from build123d import *

# Parameters (mm, degrees)
BOSS_EXTRUDE1_DEPTH  = 2.9
SOLENOID_PLACEMENT_W = 37.4
SOLENOID_PLACEMENT_H = 63.8
CUT_EXTRUDE1_DEPTH   = 103.571487266
CUT_EXTRUDE3_DEPTH   = 103.571487266
SKETCH4_W            = 13
SKETCH4_H            = 26.3
CUT_EXTRUDE4_DEPTH   = 98.286484159
CUT_EXTRUDE5_DEPTH   = 98.286484159
SKETCH6_R            = 2.25
CUT_EXTRUDE6_DEPTH   = 98.286484159


with BuildPart() as part:
    # Sketch1 → Boss-Extrude1 (new body)
    with BuildSketch(Plane(origin=(0, 0, 0), x_dir=(1, 0, 0), z_dir=(0, 1, 0))):
        with BuildLine():
            ThreePointArc((33.29110537, -64.404598464), (0, 72.5), (-33.29110537, -64.404598464))
            ThreePointArc((-33.29110537, -64.404598464), (0, -44.989799638), (33.29110537, -64.404598464))
        make_face()
    extrude(amount=BOSS_EXTRUDE1_DEPTH)

    # solenoid placement → Cut-Extrude1 (cut, through all)
    with BuildSketch(Plane(origin=(0, 2.9, 0), x_dir=(1, 0, 0), z_dir=(0, 1, 0))):
        with Locations((0, -3.8)):
            Rectangle(SOLENOID_PLACEMENT_W, SOLENOID_PLACEMENT_H)
    extrude(amount=-CUT_EXTRUDE1_DEPTH, mode=Mode.SUBTRACT)

    # Sketch3 → Cut-Extrude3 (cut, through all)
    with BuildSketch(Plane(origin=(0, 2.9, 0), x_dir=(1, 0, 0), z_dir=(0, 1, 0))):
        with BuildLine():
            Line((-34.63, -32.5), (-22.83, -32.5))
            Line((-22.83, -32.5), (-22.83, 32.5))
            Line((-22.83, 32.5), (-64.807406984, 32.5))
            ThreePointArc((-64.807406984, 32.5), (-72.5, 0), (-64.807406984, -32.5))
            Line((-64.807406984, -32.5), (-34.63, -32.5))
        make_face()
        with BuildLine():
            Line((34.63, -32.5), (64.807406984, -32.5))
            ThreePointArc((64.807406984, -32.5), (72.5, 0), (64.807406984, 32.5))
            Line((64.807406984, 32.5), (22.83, 32.5))
            Line((22.83, 32.5), (22.83, -32.5))
            Line((22.83, -32.5), (34.63, -32.5))
        make_face()
    extrude(amount=-CUT_EXTRUDE3_DEPTH, mode=Mode.SUBTRACT)

    # Sketch4 → Cut-Extrude4 (cut, through all)
    with BuildSketch(Plane(origin=(0, 2.9, 0), x_dir=(1, 0, 0), z_dir=(0, 1, 0))):
        with Locations((0, 41.25)):
            Rectangle(SKETCH4_W, SKETCH4_H)
    extrude(amount=-CUT_EXTRUDE4_DEPTH, mode=Mode.SUBTRACT)

    # Sketch5 → Cut-Extrude5 (cut, through all)
    with BuildSketch(Plane(origin=(0, 2.9, 0), x_dir=(1, 0, 0), z_dir=(0, 1, 0))):
        Polygon((-18.706882066, 48), (-21.853441033, 53.45), (-28.146558967, 53.45), (-31.293117934, 48), (-28.146558967, 42.55), (-21.853441033, 42.55), align=None)
        Polygon((21.853441033, 42.55), (18.706882066, 48), (21.853441033, 53.45), (28.146558967, 53.45), (31.293117934, 48), (28.146558967, 42.55), align=None)
    extrude(amount=-CUT_EXTRUDE5_DEPTH, mode=Mode.SUBTRACT)

    # Sketch6 → Cut-Extrude6 (cut, through all)
    with BuildSketch(Plane(origin=(0, 2.9, 0), x_dir=(1, 0, 0), z_dir=(0, 1, 0))):
        with Locations(Location((35, -50, 0), (0, 0, 270))):
            Circle(SKETCH6_R)
        with Locations(Location((-35, -50, 0), (0, 0, 270))):
            Circle(SKETCH6_R)
        with Locations(Location((-50, 40, 0), (0, 0, 270))):
            Circle(SKETCH6_R)
        with Locations(Location((50, 40, 0), (0, 0, 270))):
            Circle(SKETCH6_R)
    extrude(amount=-CUT_EXTRUDE6_DEPTH, mode=Mode.SUBTRACT)


solid = part.part
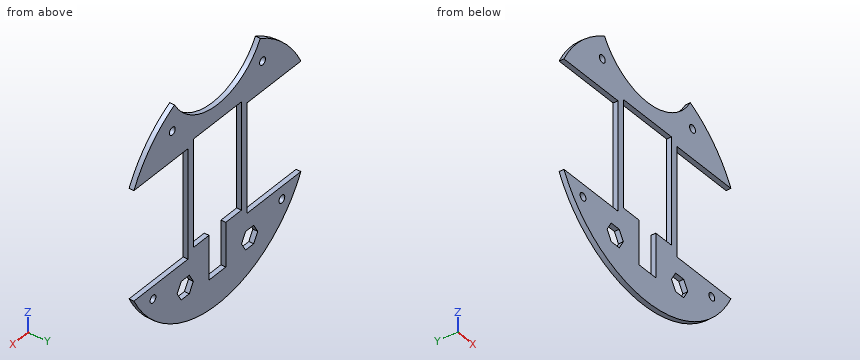
Verification items for the finished model (mm, model axes). Round coordinates to 2 decimals unless told otherwise and drop trailing zeros. Order: outer loops, then holes, each group sorted by start corner. A loop starts at its lowest first (then second) coordinate and runs counter-clockwise, first axis right, second up.
1. Section check C-C on y = 2.35. State how many separate pieces and enclosed holes the cut face has, then the cut area to 3 significant figures.
Final values:
separate pieces: 1
enclosed holes: 7
area: 6,100 mm2
2. Section check D-D on z = 50. Record the cut outline in (x, y), then the cut area to 3 significant figures.
Final values:
outline: (-52.5, 0) - (-37.25, 0) - (-37.25, 2.9) - (-52.5, 2.9) - close; (-32.75, 0) - (-18.93, 0) - (-18.93, 2.9) - (-32.75, 2.9) - close; (18.93, 0) - (32.75, 0) - (32.75, 2.9) - (18.93, 2.9) - close; (37.25, 0) - (52.5, 0) - (52.5, 2.9) - (37.25, 2.9) - close
area: 169 mm2
3. Go/stop test with flat-tipped pins: P1, Ø1.4, axis at x = 1.5, y = 2, coming from the +Z side; P2, Ø2.5, axis at x = -50, z = -40, coming from the -Y side; P3, Ø1.4, axis at y = 2, z = -7, coming from the +X side; P4, Ø1.4, axis at x = 26, y = 2, coming from the +Z side. Record where each tip stops, or that it passes through.
Final values:
P1: stops at z = 45.05
P2: passes through
P3: stops at x = 22.83
P4: stops at z = 55.85
4. Thickness scan on L1, parallel to X at y = 0.7, z = -40; L2, parallel to X at y = 1.9, z = 0.5; L3, parallel to Z at x = 48, y = 2. Record the ranges inside material, lowest first.
Final values:
L1: x = -60.47 to -52.25, -47.75 to -6.5, 6.5 to 47.75, 52.25 to 60.47
L2: x = -22.83 to -18.7, 18.7 to 22.83
L3: z = -54.33 to -41.03, -38.97 to -32.5, 32.5 to 54.33
5. Section check B-B on z = -25. Record the cut outline in (x, y), then the cut area to 3 significant figures.
Final values:
outline: (-22.83, 0) - (-18.7, 0) - (-18.7, 2.9) - (-22.83, 2.9) - close; (18.7, 0) - (22.83, 0) - (22.83, 2.9) - (18.7, 2.9) - close
area: 24.0 mm2
6. Section check A-A on x = -50. Record the cut outline in (y, z).
Final values:
outline: (0, -52.5) - (2.9, -52.5) - (2.9, -42.25) - (0, -42.25) - close; (0, -37.75) - (2.9, -37.75) - (2.9, -32.5) - (0, -32.5) - close; (0, 32.5) - (2.9, 32.5) - (2.9, 52.5) - (0, 52.5) - close
